Design review of the part built by this model. Coordinates are the model's own, in mm. A direction names the side the tool comes from. Round coordinates to 2 decimals unless told otherwise and drop trailing zeros. Loops run counter-clockwise (first coordinate to the right, second up) from the corner with the lowest first, then second, coordinate; pieces in that order, holes last. Notation, with made-up numbers: (-39, -2.5) -> (-23, -2.5) arc R10 cw to (-23, 14.5) -> close; hole circle Ø5 at (86.25, 15.25). An arc over 180 degrees is marked (long way). Answer as CSV lines item,"result". Start each with the question number.
```python
from build123d import *

# Parameters (mm, degrees)
BOSS_EXTRUDE1_DEPTH = 30
SKETCH3_R           = 4.1
CUT_EXTRUDE1_DEPTH  = 81.160460929
SKETCH4_R           = 4.1
CUT_EXTRUDE2_DEPTH  = 72.938334134
FILLET1_R           = 7
BOSS_EXTRUDE2_DEPTH = 30
SKETCH7_R           = 4.1
CUT_EXTRUDE3_DEPTH  = 154.802223385
SKETCH8_W           = 10
SKETCH8_H           = 50
CUT_EXTRUDE4_DEPTH  = 151.209521461


with BuildPart() as part:
    # Sketch1 → Boss-Extrude1 (new body)
    with BuildSketch(Plane(origin=(0, 0, 0), x_dir=(1, 0, 0), z_dir=(0, 1, 0))):
        Polygon((-22.986013986, 8.601398601), (-22.986013986, -11.398601399), (-5.986013986, -11.398601399), (-5.986013986, -2.307692308), (8.013986014, -2.307692308), (8.013986014, -11.398601399), (25.013986014, -11.398601399), (25.013986014, 8.601398601), (6.013986014, 8.601398601), (6.013986014, 58.601398601), (-3.986013986, 58.601398601), (-3.986013986, 8.601398601), align=None)
    extrude(amount=BOSS_EXTRUDE1_DEPTH)

    # Sketch3 → Cut-Extrude1 (cut, through all)
    with BuildSketch(Plane.XY.offset(11.398601399)):
        with Locations((-14.486013986, 15)):
            Circle(SKETCH3_R)
        with Locations((16.513986014, 15)):
            Circle(SKETCH3_R)
    extrude(amount=-CUT_EXTRUDE1_DEPTH, mode=Mode.SUBTRACT)

    # Sketch4 → Cut-Extrude2 (cut, through all)
    with BuildSketch(Plane(origin=(6.013986014, 0, 0), x_dir=(0, 0, -1), z_dir=(1, 0, 0))):
        with Locations((28.601398601, 15)):
            Circle(SKETCH4_R)
        with Locations((48.601398601, 15)):
            Circle(SKETCH4_R)
    extrude(amount=-CUT_EXTRUDE2_DEPTH, mode=Mode.SUBTRACT)

    # Fillet1
    fillet1_edges = [part.edges().sort_by_distance(p)[0] for p in [
        (-5.986013986, 15, 2.307692308),
        (8.013986014, 15, 2.307692308),
    ]]
    fillet(fillet1_edges, radius=FILLET1_R - 0.0001)  # a hair under: the kernel refuses the full size

    # Sketch6 → Boss-Extrude2 (add)
    with BuildSketch(Plane.XZ):
        Polygon((25.013986014, 11.398601399), (135.013986014, 11.398601399), (135.013986014, -58.601398601), (115.013986014, -58.601398601), (115.013986014, -8.601398601), (25.013986014, -8.601398601), align=None)
    extrude(amount=-BOSS_EXTRUDE2_DEPTH)

    # Sketch7 → Cut-Extrude3 (cut, through all)
    with BuildSketch(Plane.ZY.offset(3.986013986)):
        with Locations(Location((-48.601398601, 15, 0), (0, 0, 180))):
            Circle(SKETCH7_R)
        with Locations(Location((-28.601398601, 15, 0), (0, 0, 180))):
            Circle(SKETCH7_R)
    extrude(amount=-CUT_EXTRUDE3_DEPTH, mode=Mode.SUBTRACT)

    # Sketch8 → Cut-Extrude4 (cut, through all)
    with BuildSketch(Plane(origin=(0, 30, 0), x_dir=(1, 0, 0), z_dir=(0, 1, 0))):
        with Locations((1.013986014, 33.601398601)):
            Rectangle(SKETCH8_W, SKETCH8_H)
    extrude(amount=-CUT_EXTRUDE4_DEPTH, mode=Mode.SUBTRACT)


solid = part.part
```
Q1. Mouldability with a two-part tool opening along Y and no side actions: class faces 4 (the flat face through (75, 30, -8)), 5 (the flat face through (71, 15, 11.399)), 6 (the cylindrical face through (124.874, 14.82, -24.505)), 7 (the cylindrical face through (13.26, 12.505, 1.539)) as pulls with the +Y half, pulls with the -Y half, needs draft (parallel to the pull), parting line crosses it, or undercut.
Q2. For pin 1 Ø4 at (x, z) = (78, -4) entering from -Y; pin 2 Ø9.5 at (x, y) = (-14.49, 15) entering from -Z; pin 3 Ø10.5 at (y, z) = (15, -48.6) entering from -X, all flat-tipped, find the tip position at first contact; note any pin that passes through.
Q3. Add section B-B, the plane z = -27. Give the boundary of the cut face in (x, y).
Q4. Machinability: for faces 1 (the cylindrical face through (5.909, 15.21, 4.304)), 2 (the flat face through (115.014, 15, -34)), 3 (the flat face through (135.014, 15, -23)), which of the approach directions +Z, -Z, +X, -X, +Y, -Y give a long, thin tool a straight path to every point of the face, cutting with its end or side? Answer none if there is none.
Q5. Add section A-A, the plane y = 15. State how many separate pieces and enclosed holes the cut face has, and give its area (3 significant figures).
Q6. To check wall thickness, follow probe 1 along Z at (x, y) = (121, 15); probe 2 along X at (y, z) = (21, -9.5); probe 3 along Z at (x, y) = (64, 24). State the ranges of each line that lie inside material, in increasing order. Write a range as from..to.
Q7. Add section C-C, the plane x = 18.5. Give the boundary of the cut face in (y, z), and give its area (3 significant figures).
Worked answers:
1,face 4,"pulls with the +Y half"
1,face 5,"needs draft"
1,face 6,"undercut"
1,face 7,"undercut"
2,pin 1,"stops at y = 0"
2,pin 2,"stops at z = -8.6"
2,pin 3,"stops at x = 115.01"
3,outline,"(115.01, 0) -> (135.01, 0) -> (135.01, 11.23) -> (115.01, 11.23) -> close; (115.01, 18.77) -> (135.01, 18.77) -> (135.01, 30) -> (115.01, 30) -> close"
4,face 1,"+Z, +Y, -Y"
4,face 2,"-Z, -X, +Y, -Y"
4,face 3,"+Z, -Z, +X, +Y, -Y"
5,separate pieces,"5"
5,enclosed holes,"0"
5,area,"3,400 mm^2"
6,probe 1,"z = -58.6..-52.7, -44.5..-32.7, -24.5..11.4"
6,probe 2,"x = 115.01..135.01"
6,probe 3,"z = -8.6..11.4"
7,outline,"(0, -8.6) -> (11.41, -8.6) -> (11.41, 11.4) -> (0, 11.4) -> close; (18.59, -8.6) -> (30, -8.6) -> (30, 11.4) -> (18.59, 11.4) -> close"
7,area,"457 mm^2"
